Verification items for the finished model (mm, model axes). Face numbers are marked on the shaded views. A direction names the side the tool comes from. Give positions to 0.01 mm unless a question says otherwise; leave off trailing zeros. Answer as a JSON object with one key per item and string values.
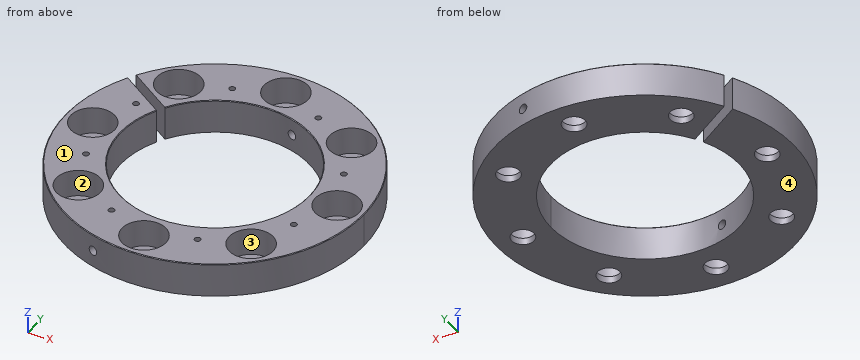
```python
from build123d import *

# Parameters (mm, degrees)
SKETCH2_R                                 = 56.134
BOSS_EXTRUDE1_DEPTH                       = 12.7
SKETCH3_R                                 = 35.433
CUT_EXTRUDE1_DEPTH                        = 13.7
CHAMFER1_SIZE                             = 0.254
CBORE_FOR_5_16_HEX_HEAD_BOLT2_D           = 8.4328
CBORE_FOR_5_16_HEX_HEAD_BOLT2_CBORE_D     = 16.51
CBORE_FOR_5_16_HEX_HEAD_BOLT2_CBORE_DEPTH = 10.16
CIRPATTERN1_COUNT                         = 8
CIRPATTERN2_COUNT                         = 8
CUT_EXTRUDE2_DEPTH                        = 13.7
F_8_32_TAPPED_HOLE2_D                     = 3.4544


with BuildPart() as part:
    # Sketch2 → Boss-Extrude1 (new body)
    with BuildSketch(Plane.XY):
        Circle(SKETCH2_R)
    extrude(amount=BOSS_EXTRUDE1_DEPTH)

    # Sketch3 → Cut-Extrude1 (cut, through all)
    with BuildSketch(Plane.XY.offset(12.7)):
        Circle(SKETCH3_R)
    extrude(amount=-CUT_EXTRUDE1_DEPTH, mode=Mode.SUBTRACT)

    # Chamfer1
    chamfer1_edges = [part.edges().sort_by_distance(p)[0] for p in [
        (-56.134, 0, 12.7),
        (-35.433, 0, 12.7),
    ]]
    chamfer(chamfer1_edges, length=CHAMFER1_SIZE)

    # CBORE for 5_16 Hex Head Bolt2 (through all)
    with Locations(Plane.XY.offset(12.7)):
        with Locations((0, 46.0756)):
            cbore_for_5_16_hex_head_bolt2 = CounterBoreHole(CBORE_FOR_5_16_HEX_HEAD_BOLT2_D / 2, CBORE_FOR_5_16_HEX_HEAD_BOLT2_CBORE_D / 2, CBORE_FOR_5_16_HEX_HEAD_BOLT2_CBORE_DEPTH)

    # CirPattern1: CBORE for 5_16 Hex Head Bolt2 ×8 about axis
    cirpattern1_axis = Axis((0, 0, 0), (0, 0, 1))
    for i in range(1, CIRPATTERN1_COUNT):
        add(cbore_for_5_16_hex_head_bolt2.rotate(cirpattern1_axis, i * 360 / CIRPATTERN1_COUNT), mode=Mode.SUBTRACT)

    # Sketch21 → 4-40 Tapped Hole1 (revolve, cut)
    with BuildSketch(Plane(origin=(-16.232665834, 39.18912201, 12.7), x_dir=(0, -1, 0), z_dir=(1, 0, 0))):
        Polygon((0, 0), (0, 8.273752758), (1.1303, 7.5946), (1.1303, 0), align=None)
    f_4_40_tapped_hole1 = revolve(axis=Axis((-16.232665834, 39.18912201, 19.05), (0, 0, -1)), mode=Mode.SUBTRACT)

    # CirPattern2: 4-40 Tapped Hole1 ×8 about axis
    cirpattern2_axis = Axis((0, 0, 0), (0, 0, 1))
    for i in range(1, CIRPATTERN2_COUNT):
        add(f_4_40_tapped_hole1.rotate(cirpattern2_axis, i * 360 / CIRPATTERN2_COUNT), mode=Mode.SUBTRACT)

    # Sketch26 → Cut-Extrude2 (cut, through all)
    with BuildSketch(Plane.XY.offset(12.7)):
        Polygon((0, 0), (-58.152698702, 37.047354929), (-59.858624959, 34.369587088), (-1.705926257, -2.67776784), align=None)
    extrude(amount=-CUT_EXTRUDE2_DEPTH, mode=Mode.SUBTRACT)

    # 8-32 Tapped Hole2 (through all)
    with Locations(Plane(origin=(14.528548278, 54.221280333, 6.35), x_dir=(0.965925826, -0.258819045, 0), z_dir=(0.258819045, 0.965925826, 0))):
        with Locations((0, 0)):
            Hole(F_8_32_TAPPED_HOLE2_D / 2)


solid = part.part
```
1) Section check A-A on z = 10.25. Count the separate pieces of the cut face and the enclosed holes in it, and give its area (3 significant figures).
Completed:
{"separate pieces": "1", "enclosed holes": "16", "area": "4,140 mm2"}
2) Access from +Z, -Z, +X, -X, +Y, -Y to the whole of each face (thin tool, end or side, straight path). Record for the marked faces 3 and 4.
Completed:
{"face 3": "+Z", "face 4": "-Z, +X, -X, +Y, -Y"}
3) Thickness scan on L1, parallel to X at y = 0, z = 5.25; L2, parallel to X at y = 16.5, z = 7.75; L3, parallel to Y at x = 2, z = 8. Record the ranges inside material, lowest first.
Completed:
{"L1": "x = -56.13 to -54.33, -37.82 to -35.43, 35.43 to 37.82, 54.33 to 56.13", "L2": "x = -53.65 to -40.29, -38.09 to -31.81, 31.36 to 38.09, 40.29 to 53.65", "L3": "y = -56.1 to -54.08, -38.07 to -35.38, 35.38 to 38.07, 54.08 to 56.1"}
4) Release check for a two-part mould opening along Y. For the marked faces 1 and 2 record: pulls with the +Y half, pulls with the -Y half, needs draft (parallel to the pull), parting line crosses it, or undercut.
Completed:
{"face 1": "needs draft", "face 2": "undercut"}
5) Go/stop test with flat-tipped pins: pin 1 (2 mm diameter, centred on y = -12, z = 8.5, fed in from -X); pin 2 (11 mm diameter, centred on x = 32.58, y = 32.58, fed in from +Z); pin 3 (2 mm diameter, centred on y = 7, z = 2.5, fed in from -X). Record where each tip stops, or that it passes through.
Completed:
{"pin 1": "stops at x = -55.05", "pin 2": "stops at z = 2.54", "pin 3": "stops at x = -55.81"}
